Print and shaded views of the part. All mm, measured from the part's lowest x, y and z. A direction names the side the tool comes from. Round coordinates to 2 decimals unless told otherwise and drop trailing zeros. Loops run counter-clockwise (first coordinate to the right, second up) from the corner with the lowest first, then second, coordinate; pieces in that order, holes last. Notation, with made-up numbers: (-38.75, 61.5) - (2.25, 61.5) arc R12 cw to (2.25, 74.5) - close; hole circle Ø2 at (64, 13). An arc over 180 degrees is marked (long way). Use one line per item in the form item = value. Start each with the question number.
Q1. Drill centre lines: line 1 (Y direction, x = 6.35, z = 12.25); line 2 (Z direction, x = 8.5, y = 7.25) (3 decimals); line 3 (Y direction, x = 5.5, z = 18). Where is each one in solid material? Low to high.
Q2. Saw through at A-A (z = 3). Give the cut face in (x, y).
Q3. Saw through at B-B (y = 10.5). Give the cut face in (x, z).
Q4. Mould opens along X. For the marked faces 1, 2 and 3 say: released by +X, released by -X, zero draft, split by the parting line, or undercut.
Q5. 3-axis set-ups, long thin cutter, end or side, ignore diameter. For the marked faces 4 and 5: which of +Z, -Z, +X, -X, +Y, -Y reach the whole face in a straight line?
Q6. Saw through at D-D (y = 1). Give the cut face in (x, z).
Q7. Saw through at C-C (x = 9.75). Give the cut face in (y, z).
Q8. Pin check, flat tips, straight feed: pin 1 (1.5 mm diameter, centred on x = 7, y = 7, fed in from -Z) (3 decimals); pin 2 (1 mm diameter, centred on y = 8, z = 14, fed in from +X); pin 3 (4 mm diameter, centred on x = 1.5, z = 21.5, fed in from +Y). Stop position of each tip, or through.
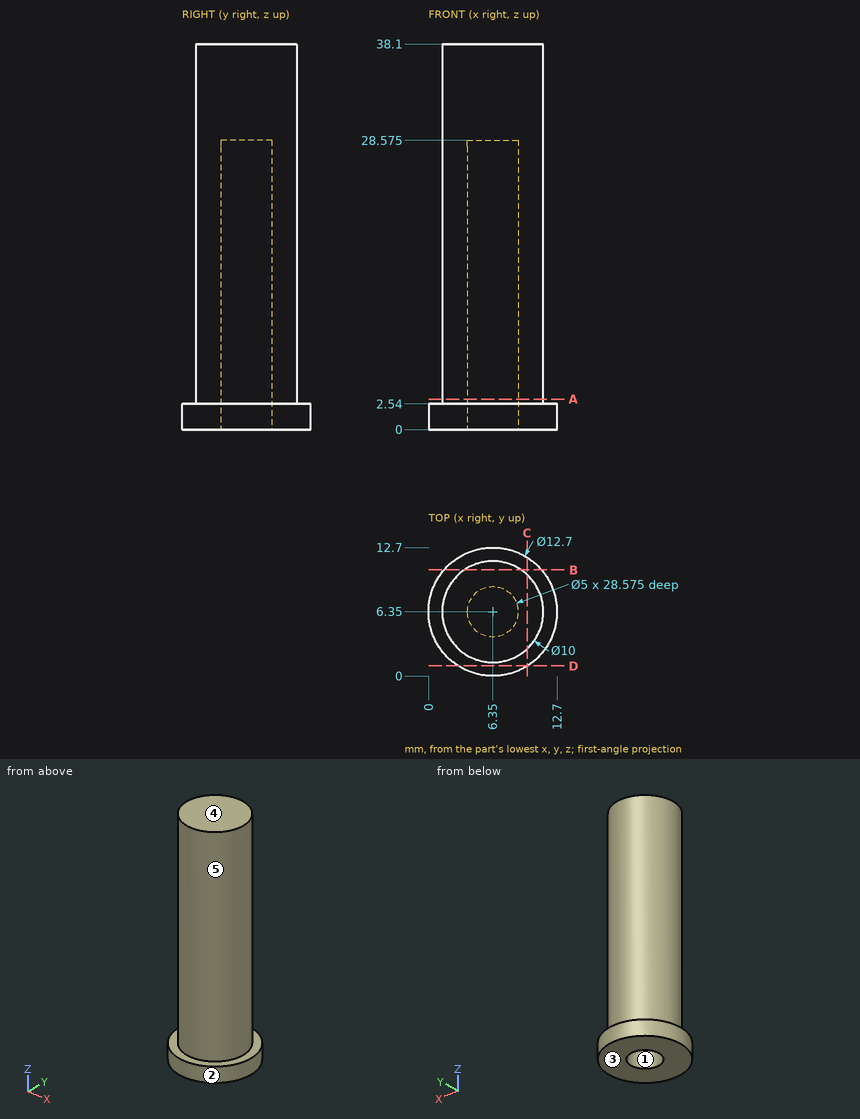
Report:
q1.line_1 = 1.35 to 3.85, 8.85 to 11.35
q1.line_2 = 28.575 to 38.1
q1.line_3 = 1.42 to 4, 8.7 to 11.28
q2.outline = circle Ø10 at (6.35, 6.35); hole circle Ø5 at (6.35, 6.35)
q3.outline = (1.54, 0) - (11.16, 0) - (11.16, 2.54) - (9.14, 2.54) - (9.14, 38.1) - (3.56, 38.1) - (3.56, 2.54) - (1.54, 2.54) - close
q4.face_1 = undercut
q4.face_2 = split by the parting line
q4.face_3 = zero draft
q5.face_4 = +Z, +X, -X, +Y, -Y
q5.face_5 = +Z
q6.outline = (2.93, 0) - (9.77, 0) - (9.77, 2.54) - (2.93, 2.54) - close
q7.outline = (0.99, 0) - (11.71, 0) - (11.71, 2.54) - (10.02, 2.54) - (10.02, 38.1) - (2.68, 38.1) - (2.68, 2.54) - (0.99, 2.54) - close
q8.pin_1 = 28.575
q8.pin_2 = 11.22
q8.pin_3 = 10.46
